Can you work these out from the model? Positions are in its coordinate system, mm. Face numbers are marked on the shaded views. A direction names the side the tool comes from. Give positions to 0.01 mm unless a question says otherwise; leave off trailing zeros. Order: outer loops, then holes, each group sorted by start corner. A loop starts at its lowest first (then second) coordinate and runs counter-clockwise, first axis right, second up. Notation, with made-up numbers: (-36.5, 51.5) - (20.5, 51.5) arc R25 cw to (20.5, 88.5) - close; hole circle Ø3 at (11, 3.25). An arc over 180 degrees is marked (long way). Return JSON: item names as keys, results as strings.
```python
from build123d import *

# Parameters (mm, degrees)
SKETCH1_W           = 40
SKETCH1_H           = 25
SKETCH1_R           = 3.1
BOSS_EXTRUDE1_DEPTH = 3
SKETCH2_W           = 3
SKETCH2_H           = 25
BOSS_EXTRUDE2_DEPTH = 40
SKETCH3_R           = 3.1
CUT_EXTRUDE1_DEPTH  = 60.949979149
BOSS_EXTRUDE3_DEPTH = 10


with BuildPart() as part:
    # Sketch1 → Boss-Extrude1 (new body)
    with BuildSketch(Plane(origin=(0, 0, 0), x_dir=(1, 0, 0), z_dir=(0, 1, 0))):
        with Locations((20, -12.5)):
            Rectangle(SKETCH1_W, SKETCH1_H)
        with Locations(Location((10, -12.5, 0), (0, 0, 270))):
            Circle(SKETCH1_R, mode=Mode.SUBTRACT)
    extrude(amount=BOSS_EXTRUDE1_DEPTH)

    # Sketch2 → Boss-Extrude2 (add)
    with BuildSketch(Plane.XZ):
        with Locations((38.5, 12.5)):
            Rectangle(SKETCH2_W, SKETCH2_H)
    extrude(amount=BOSS_EXTRUDE2_DEPTH)

    # Sketch3 → Cut-Extrude1 (cut, through all)
    with BuildSketch(Plane.ZY.offset(-37)):
        with Locations((12.5, -27)):
            Circle(SKETCH3_R)
    extrude(amount=-CUT_EXTRUDE1_DEPTH, mode=Mode.SUBTRACT)

    # Sketch4 → Boss-Extrude3 (add, symmetric)
    with BuildSketch(Plane.XY.offset(12.5)):
        Polygon((15.275287554, 0), (37, -23.590932737), (37, 0), align=None)
    extrude(amount=BOSS_EXTRUDE3_DEPTH, both=True)


solid = part.part
```
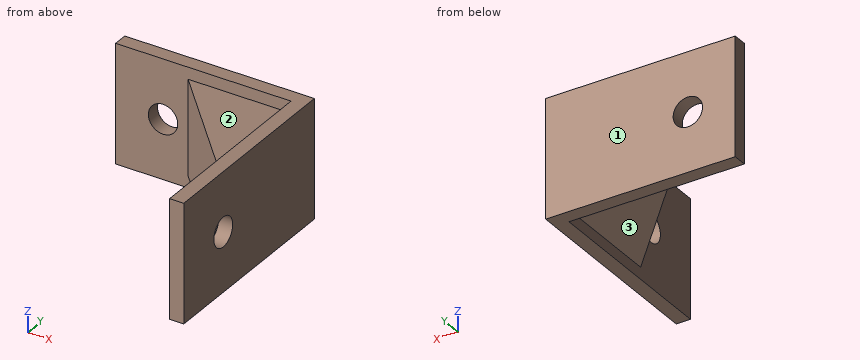
1. On a 3-axis mill with a long thin cutter (end or side, diameter ignored), from which of +Z, -Z, +X, -X, +Y, -Y can I reach the whole of each face in a straight line? I mean the marked faces 1, 2 and 3. Say none if no direction works.
Checks:
{"face 1": "+Z, -Z, +X, -X, +Y", "face 2": "+Z, -X, -Y", "face 3": "-Z, -X, -Y"}
2. If I drill on L1, parallel to X at y = 2.05, z = 12.5; L2, parallel to Y at x = 38.9, z = 12.5; L3, parallel to X at y = -29, z = 23, over which ranges is the centre line in solid material (lowest first)? Write a range as [from, to].
Checks:
{"L1": "[0, 6.9], [13.1, 40]", "L2": "[-40, -30.1], [-23.9, 3]", "L3": "[37, 40]"}
3. For pin 1 Ø2 at (y, z) = (-13, 20.5) entering from -X; pin 2 Ø6.5 at (x, y) = (30.5, -7) entering from -Z; pin 3 Ø6.5 at (x, y) = (28, -9) entering from +Z, each with a flat end and sliding along its axis, tell me the tip position at first contact or that it passes through.
Checks:
{"pin 1": "x = 26.33", "pin 2": "z = 2.5", "pin 3": "z = 22.5"}
4. Suppose I cut it at D-D (z = 7.5). List the corners of the cut face in (x, y) for me.
Checks:
{"outline": "(0, 0) - (15.28, 0) - (37, -23.59) - (37, -40) - (40, -40) - (40, 3) - (0, 3) - close"}
5. Suppose I cut it at C-C (z = 12.5). List the corners of the cut face in (x, y) for me.
Checks:
{"outline": "(0, 0) - (6.9, 0) - (6.9, 3) - (0, 3) - close; (13.1, 0) - (15.28, 0) - (37, -23.59) - (37, -23.9) - (40, -23.9) - (40, 3) - (13.1, 3) - close; (37, -40) - (40, -40) - (40, -30.1) - (37, -30.1) - close"}
6. Suppose I cut it at B-B (x = 10). List the corners of the cut face in (y, z) for me, plus the area to 3 significant figures.
Checks:
{"outline": "(0, 0) - (3, 0) - (3, 9.4) - (0, 9.4) - close; (0, 15.6) - (3, 15.6) - (3, 25) - (0, 25) - close", "area": "56.4 mm^2"}
7. Suppose I cut it at A-A (y = -27). List the corners of the cut face in (x, z) for me, plus the area to 3 significant figures.
Checks:
{"outline": "(37, 0) - (40, 0) - (40, 9.4) - (37, 9.4) - close; (37, 15.6) - (40, 15.6) - (40, 25) - (37, 25) - close", "area": "56.4 mm^2"}
